Can you work these out from the model? Positions are in its coordinate system, mm. Face numbers are marked on the shaded views. A direction names the side the tool comes from. Round coordinates to 2 decimals unless told otherwise and drop trailing zeros. Order: outer loops, then holes, each group sorted by start corner. A loop starts at its lowest first (then second) coordinate and runs counter-clockwise, first axis right, second up. Notation, with made-up numbers: M -7,12.25 L 52,12.25 A21 ccw 52,36.25 Z; hole C 28,44 d11. An arc over 180 degrees is marked long. One line per question, with ' | ' between items.
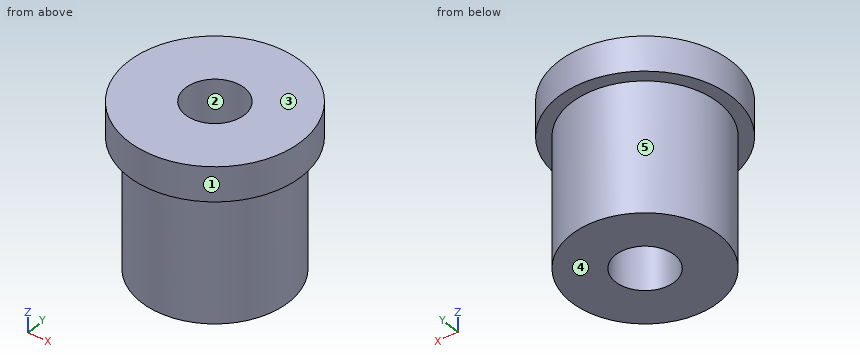
```python
from build123d import *

# Parameters (mm, degrees)
SKETCH1_R              = 10
BOSS_EXTRUDE1_DEPTH    = 4
SKETCH2_R              = 8.5
BOSS_EXTRUDE2_DEPTH    = 15
M8X1_25_TAPPED_HOLE2_D = 6.8


with BuildPart() as part:
    # Sketch1 → Boss-Extrude1 (new body)
    with BuildSketch(Plane.XY):
        Circle(SKETCH1_R)
    extrude(amount=BOSS_EXTRUDE1_DEPTH)

    # Sketch2 → Boss-Extrude2 (add)
    with BuildSketch(Plane(origin=(0, 0, 0), x_dir=(-1, 0, 0), z_dir=(0, 0, -1))):
        Circle(SKETCH2_R)
    extrude(amount=BOSS_EXTRUDE2_DEPTH)

    # M8x1.25 Tapped Hole2 (through all)
    with Locations(Plane.XY.offset(4)):
        with Locations((0, 0)):
            Hole(M8X1_25_TAPPED_HOLE2_D / 2)


solid = part.part
```
(1) If we section it at C-C on y = 5.75: Please give me the cut outline in (x, z).
Final values:
outline: M -8.18,0 L -6.26,0 L -6.26,-15 L 6.26,-15 L 6.26,0 L 8.18,0 L 8.18,4 L -8.18,4 Z
(2) Thinking about a two-plate mould opening in Y: for the marked faces 1, 2 and 3, which applies, released by +Y, released by -Y, zero draft, split by the parting line, or undercut?
Final values:
face 1: split by the parting line | face 2: undercut | face 3: zero draft
(3) Will these pins go through, and if not, where does the flat tip stop? pin 1 Ø2 at (y, z) = (4, -6.5) entering from -X; pin 2 Ø1 at (y, z) = (-4.5, -6.5) entering from +X; pin 3 Ø1 at (y, z) = (-2.5, -1) entering from -X.
Final values:
pin 1: x = -7.95 | pin 2: x = 7.5 | pin 3: x = -8.26
(4) On a 3-axis mill with a long thin cutter (end or side, diameter ignored), from which of +Z, -Z, +X, -X, +Y, -Y can I reach the whole of each face in a straight line? I mean the marked faces 4 and 5. Say none if no direction works.
Final values:
face 4: -Z, +X, -X, +Y, -Y | face 5: -Z
(5) Please list where these lines run through material, in increasing order: probe 1 along Y at (x, z) = (0, -3.5); probe 2 along X at (y, z) = (-1, -9.75); probe 3 along X at (y, z) = (-2.25, -4). Write a range as [from, to].
Final values:
probe 1: [-8.5, -3.4], [3.4, 8.5] | probe 2: [-8.44, -3.25], [3.25, 8.44] | probe 3: [-8.2, -2.55], [2.55, 8.2]
(6) If we section it at A-A on x = 0: Please give me the cut outline in (y, z).
Final values:
outline: M -10,0 L -8.5,0 L -8.5,-15 L -3.4,-15 L -3.4,4 L -10,4 Z; M 3.4,-15 L 8.5,-15 L 8.5,0 L 10,0 L 10,4 L 3.4,4 Z
(7) If we section it at D-D on z = -5.25: Please give me the cut outline in (x, y).
Final values:
outline: C 0,0 d17; hole C 0,0 d6.8
